The model under review builds one solid part; all positions refer to its coordinate system, in mm. A direction names the side the tool comes from. Give positions to 0.01 mm unless a question says otherwise; leave off trailing zeros. Loops run counter-clockwise (first coordinate to the right, second up) from the corner with the lowest first, then second, coordinate; pieces in that order, holes last. Notation, with made-up numbers: (-25, -18) - (8, -18) arc R26 ccw to (8, 2) - close; hole circle Ø10 at (5.25, 80.25). An arc over 180 degrees is marked (long way). Return JSON: item names as keys, results as strings. Group by question number.
```python
from build123d import *

# Parameters (mm, degrees)
SKETCH1_W             = 203.2
SKETCH1_H             = 127
BOSS_EXTRUDE1_DEPTH   = 50.8
SKETCH2_W             = 196.85
SKETCH2_H             = 120.65
CUT_EXTRUDE1_DEPTH    = 47.625
SKETCH4_W             = 234.95
SKETCH4_H             = 158.75
SKETCH4_W_2           = 203.2
SKETCH4_H_2           = 127
BOSS_EXTRUDE2_DEPTH   = 6.35
SKETCH7_W             = 212.4456
SKETCH7_H             = 136.2456
SKETCH7_W_2           = 203.2
SKETCH7_H_2           = 127
CUT_EXTRUDE2_DEPTH    = 2.6416
F_8_32_TAPPED_HOLE1_D = 3.4544
FILLET3_R             = 4.6228
FILLET4_R             = 9.2456
CUT_EXTRUDE5_DEPTH    = 143.875
CUT_EXTRUDE6_REACH    = 221.075
CUT_EXTRUDE7_REACH    = 221.075
SKETCH13_R            = 12.55395
FILLET5_R             = 3.175
F_6_CLEARANCE_HOLE1_D = 3.7973


with BuildPart() as part:
    # Sketch1 → Boss-Extrude1 (new body)
    with BuildSketch(Plane(origin=(0, 0, 0), x_dir=(1, 0, 0), z_dir=(0, 1, 0))):
        Rectangle(SKETCH1_W, SKETCH1_H)
    extrude(amount=BOSS_EXTRUDE1_DEPTH)

    # Sketch2 → Cut-Extrude1 (cut)
    with BuildSketch(Plane(origin=(0, 50.8, 0), x_dir=(1, 0, 0), z_dir=(0, 1, 0))):
        Rectangle(SKETCH2_W, SKETCH2_H)
    extrude(amount=-CUT_EXTRUDE1_DEPTH, mode=Mode.SUBTRACT)

    # Sketch4 → Boss-Extrude2 (add)
    with BuildSketch(Plane(origin=(0, 50.8, 0), x_dir=(1, 0, 0), z_dir=(0, 1, 0))):
        Rectangle(SKETCH4_W, SKETCH4_H)
        Rectangle(SKETCH4_W_2, SKETCH4_H_2, mode=Mode.SUBTRACT)
    extrude(amount=-BOSS_EXTRUDE2_DEPTH)

    # Sketch7 → Cut-Extrude2 (cut)
    with BuildSketch(Plane(origin=(0, 50.8, 0), x_dir=(1, 0, 0), z_dir=(0, 1, 0))):
        Rectangle(SKETCH7_W, SKETCH7_H)
        Rectangle(SKETCH7_W_2, SKETCH7_H_2, mode=Mode.SUBTRACT)
    extrude(amount=-CUT_EXTRUDE2_DEPTH, mode=Mode.SUBTRACT)

    # #8-32 Tapped Hole1 (through all)
    with Locations(Plane(origin=(0, 50.8, 0), x_dir=(1, 0, 0), z_dir=(0, 1, 0))):
        with Locations((55.92445, 73.7489), (111.8489, 73.7489), (111.8489, 24.582966667), (0, 73.7489), (111.8489, -24.582966667), (111.8489, -73.7489), (55.92445, -73.7489), (0, -73.7489), (-55.92445, -73.7489), (-111.8489, -73.7489), (-111.8489, -24.582966667), (-111.8489, 24.582966667), (-111.8489, 73.7489), (-55.92445, 73.7489)):
            Hole(F_8_32_TAPPED_HOLE1_D / 2)

    # Fillet3
    fillet3_edges = [part.edges().sort_by_distance(p)[0] for p in [
        (-101.6, 49.4792, -63.5),
        (101.6, 49.4792, -63.5),
        (101.6, 49.4792, 63.5),
        (-101.6, 49.4792, 63.5),
    ]]
    fillet(fillet3_edges, radius=FILLET3_R)

    # Fillet4
    fillet4_edges = [part.edges().sort_by_distance(p)[0] for p in [
        (-106.2228, 49.4792, -68.1228),
        (106.2228, 49.4792, -68.1228),
        (106.2228, 49.4792, 68.1228),
        (-106.2228, 49.4792, 68.1228),
    ]]
    fillet(fillet4_edges, radius=FILLET4_R)

    # Sketch10 → Cut-Extrude5 (cut, through all)
    with BuildSketch(Plane.XY.offset(63.5)):
        with BuildLine():
            ThreePointArc((-70.843294161, 16.6624), (-76.2, 35.6489), (-81.556705839, 16.6624))
            Line((-81.556705839, 16.6624), (-70.843294161, 16.6624))
        make_face()
        with BuildLine():
            ThreePointArc((81.556705839, 16.6624), (76.2, 35.6489), (70.843294161, 16.6624))
            Line((70.843294161, 16.6624), (81.556705839, 16.6624))
        make_face()
        with BuildLine():
            ThreePointArc((30.756705839, 16.6624), (25.4, 35.6489), (20.043294161, 16.6624))
            Line((20.043294161, 16.6624), (30.756705839, 16.6624))
        make_face()
        with BuildLine():
            ThreePointArc((-20.043294161, 16.6624), (-25.4, 35.6489), (-30.756705839, 16.6624))
            Line((-30.756705839, 16.6624), (-20.043294161, 16.6624))
        make_face()
    extrude(amount=-CUT_EXTRUDE5_DEPTH, mode=Mode.SUBTRACT)

    # Sketch12 → Cut-Extrude6 (cut, up to next)
    with BuildSketch(Plane(origin=(101.6, 0, 0), x_dir=(0, 0, -1), z_dir=(1, 0, 0)), mode=Mode.PRIVATE) as cut_extrude6_sk1:
        with BuildLine():
            ThreePointArc((-20.043294161, 16.6624), (-25.4, 35.6489), (-30.756705839, 16.6624))
            Line((-30.756705839, 16.6624), (-20.043294161, 16.6624))
        make_face()
    cut_extrude6_tool1 = extrude(cut_extrude6_sk1.sketch, amount=-CUT_EXTRUDE6_REACH, mode=Mode.PRIVATE) & part.part
    add(cut_extrude6_tool1.solids().sort_by_distance((101.6, 25.721198, 25.4))[0], mode=Mode.SUBTRACT)
    # Sketch12 → Cut-Extrude6 (cut, up to next)
    with BuildSketch(Plane(origin=(101.6, 0, 0), x_dir=(0, 0, -1), z_dir=(1, 0, 0)), mode=Mode.PRIVATE) as cut_extrude6_sk2:
        with BuildLine():
            ThreePointArc((30.756705839, 16.6624), (25.4, 35.6489), (20.043294161, 16.6624))
            Line((20.043294161, 16.6624), (30.756705839, 16.6624))
        make_face()
    cut_extrude6_tool2 = extrude(cut_extrude6_sk2.sketch, amount=-CUT_EXTRUDE6_REACH, mode=Mode.PRIVATE) & part.part
    add(cut_extrude6_tool2.solids().sort_by_distance((101.6, 25.721198, -25.4))[0], mode=Mode.SUBTRACT)

    # Sketch13 → Cut-Extrude7 (cut, up to next)
    with BuildSketch(Plane.ZY.offset(101.6), mode=Mode.PRIVATE) as cut_extrude7_sk1:
        with Locations((12.7, 25.4)):
            Circle(SKETCH13_R)
    cut_extrude7_tool1 = extrude(cut_extrude7_sk1.sketch, amount=-CUT_EXTRUDE7_REACH, mode=Mode.PRIVATE) & part.part
    add(cut_extrude7_tool1.solids().sort_by_distance((-101.6, 25.4, 12.7))[0], mode=Mode.SUBTRACT)

    # Fillet5
    fillet5_edges = [part.edges().sort_by_distance(p)[0] for p in [
        (-98.425, 26.9875, -60.325),
        (98.425, 26.9875, -60.325),
        (98.425, 26.9875, 60.325),
        (-98.425, 26.9875, 60.325),
    ]]
    fillet(fillet5_edges, radius=FILLET5_R)

    # #6 Clearance Hole1 (through all)
    with Locations(Plane(origin=(0, 44.45, 0), x_dir=(-1, 0, 0), z_dir=(0, -1, 0))):
        with Locations((-98.425, 73.7489), (-98.425, -73.7489), (98.425, -73.7489), (98.425, 73.7489)):
            Hole(F_6_CLEARANCE_HOLE1_D / 2)


solid = part.part
```
1) We need section A-A, the plane x = 76.2. Write out the cut boundary in (y, z) (3 decimals).
2) Tool access review of faces 1 (the face through (25.772, 35.642, -61.89)), 2 (the face through (-1, 22, 63.5)), 3 (the face through (-100.21, 49.46, 62.18)): name each direction out of +Z, -Z, +X, -X, +Y, -Y from which nothing blocks a thin tool from reaching the whole face with its end or side.
3) We need section D-D, the plane z = -9. Write out the cut boundary in (x, y) (3 decimals).
4) We need section C-C, the plane y = 40.5. Write out the cut boundary in (x, z) (3 decimals).
5) For pin 1 Ø1 at (x, y) = (89.5, 28.5) entering from +Z; pin 2 Ø1.5 at (x, y) = (-76, 18) entering from -Z; pin 3 Ø8 at (x, z) = (-90.5, 9.5) entering from -Y; pin 4 Ø5 at (y, z) = (36, 2) entering from -X, all flat-tipped, find the tip position at first contact; note any pin that passes through.
6) We need section B-B, the plane z = 12.7. Write out the cut boundary in (x, y) (3 decimals), plus the area to 3 significant figures.
7) Draft analysis for pull direction Y (two halves, no side actions). For faces 4 (the face through (-98.425, 33, 1)), 5 (the face through (-25.028, 35.642, -61.89)), 6 (the face through (-9, 50.8, 70)), 7 (the face through (-1, 0, -1)), state which applies: +Y half, -Y half, draft (parallel to the pull), parting line (faces both ways), or undercut.
8) To check wall thickness, follow line 1 (X direction, y = 25, z = 61); line 2 (X direction, y = 12.5, z = -54) (3 decimals); line 3 (Z direction, x = 38, y = 16.5) (3 decimals). State the ranges of each line that lie inside material, in increasing order.
Findings:
{
 "1": {"outline": "(0, -63.5) - (16.662, -63.5) - (16.662, -60.325) - (3.175, -60.325) - (3.175, 60.325) - (16.662, 60.325) - (16.662, 63.5) - (0, 63.5) - close; (35.649, -63.5) - (44.45, -63.5) - (44.45, -79.375) - (50.8, -79.375) - (50.8, -68.123) - (48.158, -68.123) - (48.158, -63.5) - (50.8, -63.5) - (50.8, -60.325) - (35.649, -60.325) - close; (35.649, 60.325) - (50.8, 60.325) - (50.8, 63.5) - (48.158, 63.5) - (48.158, 68.123) - (50.8, 68.123) - (50.8, 79.375) - (44.45, 79.375) - (44.45, 63.5) - (35.649, 63.5) - close"},
 "2": {"face 1": "+Z, -Z", "face 2": "+Z, +X, -X, -Y", "face 3": "+Y"},
 "3": {"outline": "(-117.475, 44.45) - (-101.6, 44.45) - (-101.6, 0) - (101.6, 0) - (101.6, 44.45) - (117.475, 44.45) - (117.475, 50.8) - (106.223, 50.8) - (106.223, 48.158) - (101.6, 48.158) - (101.6, 50.8) - (98.425, 50.8) - (98.425, 3.175) - (-98.425, 3.175) - (-98.425, 50.8) - (-101.6, 50.8) - (-101.6, 48.158) - (-106.223, 48.158) - (-106.223, 50.8) - (-117.475, 50.8) - close"},
 "4": {"outline": "(-101.6, -63.5) - (101.6, -63.5) - (101.6, 63.5) - (-101.6, 63.5) - close; hole (-98.425, -57.15) arc R3.175 ccw to (-95.25, -60.325) - (95.25, -60.325) arc R3.175 ccw to (98.425, -57.15) - (98.425, 57.15) arc R3.175 ccw to (95.25, 60.325) - (-95.25, 60.325) arc R3.175 ccw to (-98.425, 57.15) - close"},
 "5": {"pin 1": "stops at z = 63.5", "pin 2": "passes through", "pin 3": "stops at y = 0", "pin 4": "stops at x = -101.6"},
 "6": {"outline": "(-117.475, 44.45) - (-101.6, 44.45) - (-101.6, 37.954) - (-98.425, 37.954) - (-98.425, 50.8) - (-101.6, 50.8) - (-101.6, 48.158) - (-106.223, 48.158) - (-106.223, 50.8) - (-117.475, 50.8) - close; (-101.6, 0) - (101.6, 0) - (101.6, 44.45) - (117.475, 44.45) - (117.475, 50.8) - (106.223, 50.8) - (106.223, 48.158) - (101.6, 48.158) - (101.6, 50.8) - (98.425, 50.8) - (98.425, 3.175) - (-98.425, 3.175) - (-98.425, 12.846) - (-101.6, 12.846) - close", "area": "1,050 mm^2"},
 "7": {"face 4": "draft", "face 5": "undercut", "face 6": "+Y half", "face 7": "-Y half"},
 "8": {"line 1": "x = -101.6 to -86.44, -65.96 to -35.64, -15.16 to 15.16, 35.64 to 65.96, 86.44 to 101.6", "line 2": "x = -101.6 to -98.425, 98.425 to 101.6", "line 3": "z = -63.5 to -60.325, 60.325 to 63.5"}
}
